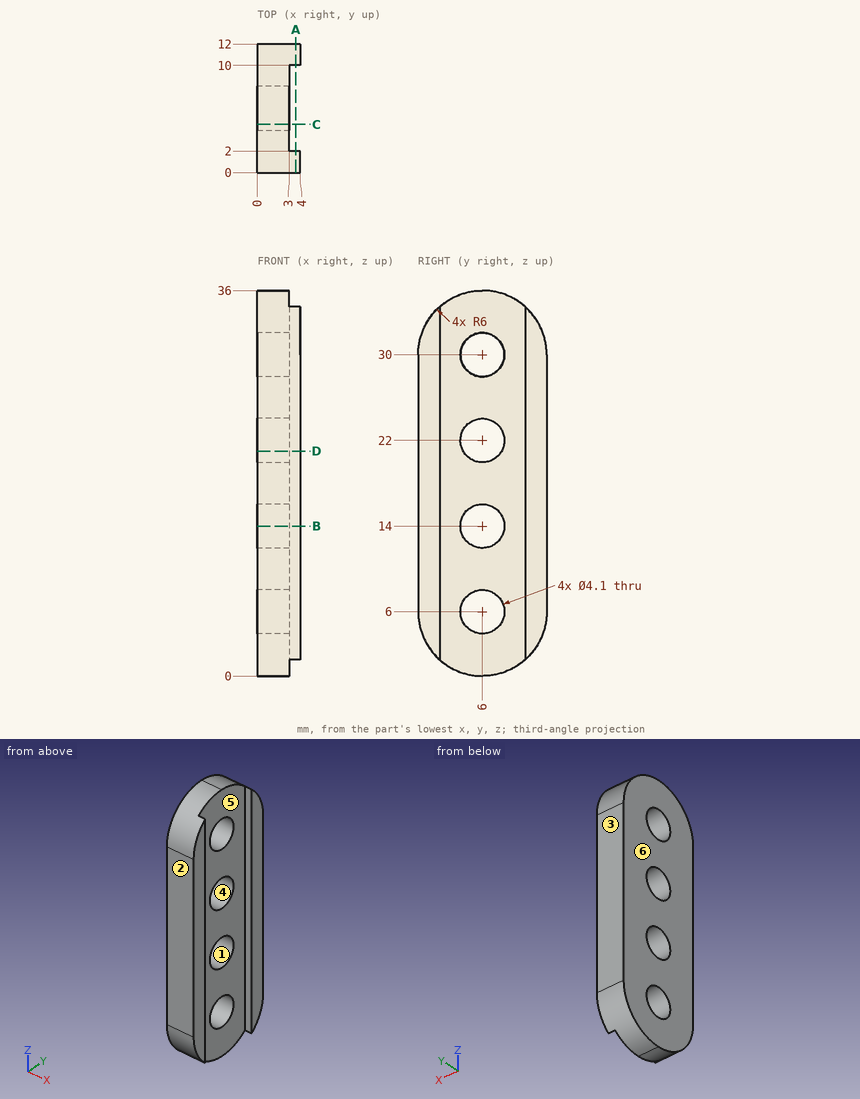
Input: dimensioned drawing with shaded views. Units: mm. Origin: part minimum x, y, z. A direction names the side the tool comes from. Coordinates: 2 decimals unless noted, no trailing zeros. Write each loop counter-clockwise with the first axis right and the second up, starting at its lowest first coordinate (ties: lowest second). Pieces come first, ordered by that corner, then holes. Notation, with made-up numbers: M 13,-4 L 24,-4 A21 cw 24,26 Z; hole C 6,64 d2. An arc over 180 degrees is marked long. Answer as a JSON object with one key per item and string values. Group by question number.
(1) Ray query, line 1 along Y through (x, z) = (0.75, 30); line 2 along X through (y, z) = (9.75, 25); line 3 along Y through (x, z) = (1.3, 31). Return the intervals inside material, ascending. Write a range as [from, to].
(2) Set-up query: the marked faces 5 and 6. Return all of +Z, -Z, +X, -X, +Y, -Y with unobstructed straight access to the full face (end or side cutting, diameter ignored); none if empty.
(3) Mould query, pull axis Y, two halves, no side actions, for the marked faces 1, 2, 3 and 4. Classes: pulls with the +Y half, pulls with the -Y half, needs draft (parallel to the pull), parting line crosses it, or undercut.
(4) Section B-B on z = 14. Output: boundary loops of the cut face in (x, y).
(5) Section A-A on x = 3.6. Output: boundary loops of the cut face in (y, z), plus the area to 3 significant figures.
(6) Section D-D on z = 21. Output: boundary loops of the cut face in (x, y), plus the area to 3 significant figures.
(7) Section C-C on y = 4.5. Output: boundary loops of the cut face in (x, z), plus the area to 3 significant figures.
(8) Contact query for flat-ended pins moving along their axis: P1, Ø6, axis at y = 9, z = 16, coming from the -X side; P2, Ø5.5, axis at y = 6, z = 22, coming from the +X side. Output: stop coordinate, or through.
Result set:
{
 "1": {"line 1": "y = [0, 3.95], [8.05, 12]", "line 2": "x = [0, 3]", "line 3": "y = [0.08, 4.21], [7.79, 11.92]"},
 "2": {"face 5": "+Z, -Z, +X", "face 6": "+Z, -Z, -X, +Y, -Y"},
 "3": {"face 1": "undercut", "face 2": "pulls with the -Y half", "face 3": "pulls with the +Y half", "face 4": "undercut"},
 "4": {"outline": "M 0,0 L 4,0 L 4,2 L 3,2 L 3,3.95 L 0,3.95 Z; M 0,8.05 L 3,8.05 L 3,10 L 4,10 L 4,12 L 0,12 Z"},
 "5": {"outline": "M 0,6 A6 ccw 2,1.53 L 2,34.47 A6 ccw 0,30 Z; M 10,1.53 A6 ccw 12,6 L 12,30 A6 ccw 10,34.47 Z", "area": "121 mm2"},
 "6": {"outline": "M 0,0 L 4,0 L 4,2 L 3,2 L 3,4.21 L 0,4.21 Z; M 0,7.79 L 3,7.79 L 3,10 L 4,10 L 4,12 L 0,12 Z", "area": "29.3 mm2"},
 "7": {"outline": "M 0,0.19 L 3,0.19 L 3,4.6 L 0,4.6 Z; M 0,7.4 L 3,7.4 L 3,12.6 L 0,12.6 Z; M 0,15.4 L 3,15.4 L 3,20.6 L 0,20.6 Z; M 0,23.4 L 3,23.4 L 3,28.6 L 0,28.6 Z; M 0,31.4 L 3,31.4 L 3,35.81 L 0,35.81 Z", "area": "73.3 mm2"},
 "8": {"P1": "stops at x = 0", "P2": "stops at x = 3"}
}
